Verification items for the finished model (mm, model axes). Face numbers are marked on the shaded views. A direction names the side the tool comes from. Round coordinates to 2 decimals unless told otherwise and drop trailing zeros. Write each loop counter-clockwise with the first axis right and the second up, starting at its lowest first coordinate (ties: lowest second). Pieces come first, ordered by that corner, then holes. Notation, with made-up numbers: (4, -1) - (49, -1) arc R28 ccw to (49, 17) - close; hole circle Ø11 at (-3.75, 4). An arc over 180 degrees is marked (long way). Answer as a JSON object with one key per item and string values. Group by question number.
1) Thickness scan on line 1 (Y direction, x = 0, z = -24.25); line 2 (Y direction, x = 3, z = -19.5); line 3 (Z direction, x = 3.5, y = -6.25). Record the ranges inside material, lowest first.
2) Section check B-B (z = 10). Enter the section's corners in (x, y).
3) Section check A-A (z = -29). Enter the section's corners in (x, y).
4) Section check C-C (x = -10.25). Enter the section's corners in (y, z), then the cut area to 3 significant figures.
5) Go/stop test with flat-tipped pins: pin 1 Ø12 at (x, z) = (-4, 14) entering from -Y; pin 2 Ø2 at (x, z) = (-1, -23.5) entering from -Y; pin 3 Ø2 at (y, z) = (2, -6) entering from +X. Record where each tip stops, or that it passes through.
6) Section check D-D (y = 8.25). Enter the section's corners in (x, z).
7) Set-up check for the marked faces 1, 2 and 3: record each of +Z, -Z, +X, -X, +Y, -Y from which the full face is reachable in a straight line by a thin tool's end or side.
```python
from build123d import *

# Parameters (mm, degrees)
SKETCH_1_R          = 6
EXTRUDE_1_DEPTH     = 20
EXTRUDE_2_DEPTH     = 6
SKETCH_3_R          = 7.5
EXTRUDE_3_DEPTH     = 1.5
SKETCH_4_R          = 5
EXTRUDE_4_DEPTH     = 26.5
SKETCH_6_R          = 6
SKETCH_6_R_2        = 5.5
CUT_EXTRUDE_1_DEPTH = 1
M5X0_8_1_D          = 4.2
M5X0_8_1_DEPTH      = 12.4
M5X0_8_1_TIP        = 1.2618073
CHAMFER_1_SIZE      = 1


with BuildPart() as part:
    # 草图1 → 凸台-拉伸1 (new body)
    with BuildSketch(Plane.XY):
        Circle(SKETCH_1_R)
    extrude(amount=EXTRUDE_1_DEPTH)

    # 草图2 → 凸台-拉伸2 (add)
    with BuildSketch(Plane(origin=(0, 0, 0), x_dir=(-1, 0, 0), z_dir=(0, 0, -1))):
        Polygon((6.350852961, 11), (-6.350852961, 11), (-12.701705922, 0), (-6.350852961, -11), (6.350852961, -11), (12.701705922, 0), align=None)
    extrude(amount=EXTRUDE_2_DEPTH)

    # 草图3 → 凸台-拉伸3 (add)
    with BuildSketch(Plane(origin=(0, 0, -6), x_dir=(-1, 0, 0), z_dir=(0, 0, -1))):
        Circle(SKETCH_3_R)
    extrude(amount=EXTRUDE_3_DEPTH)

    # 草图4 → 凸台-拉伸4 (add)
    with BuildSketch(Plane(origin=(0, 0, -7.5), x_dir=(-1, 0, 0), z_dir=(0, 0, -1))):
        Circle(SKETCH_4_R)
    extrude(amount=EXTRUDE_4_DEPTH)

    # 草图6 → 切除-拉伸1 (cut)
    with BuildSketch(Plane.XY):
        Circle(SKETCH_6_R)
        Circle(SKETCH_6_R_2, mode=Mode.SUBTRACT)
    extrude(amount=CUT_EXTRUDE_1_DEPTH, mode=Mode.SUBTRACT)

    # M5x0.8 螺纹孔1
    with Locations(Plane(origin=(0, 0, -34), x_dir=(-1, 0, 0), z_dir=(0, 0, -1))):
        with Locations((0, 0)):
            Hole(M5X0_8_1_D / 2, depth=M5X0_8_1_DEPTH)
            with Locations((0, 0, -(M5X0_8_1_DEPTH + M5X0_8_1_TIP / 2))):  # 118° drill point
                Cone(0, M5X0_8_1_D / 2, M5X0_8_1_TIP, mode=Mode.SUBTRACT)

    # 倒角1
    chamfer_1_edges = [part.edges().sort_by_distance(p)[0] for p in [
        (5, 0, -34),
        (-6, 0, 20),
    ]]
    chamfer(chamfer_1_edges, length=CHAMFER_1_SIZE)


solid = part.part
```
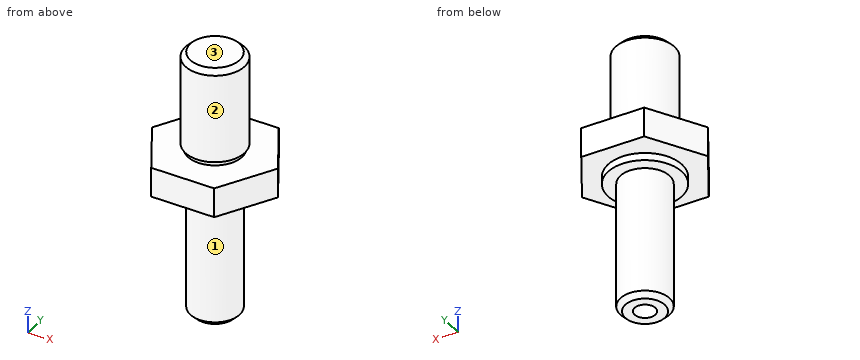
Returned:
{
 "1": {"line 1": "-5 to -2.1, 2.1 to 5", "line 2": "-4 to 4", "line 3": "-7.5 to 0"},
 "2": {"outline": "circle Ø12 at (0, 0)"},
 "3": {"outline": "circle Ø10 at (0, 0); hole circle Ø4.2 at (0, 0)"},
 "4": {"outline": "(-4.25, -6) - (4.25, -6) - (4.25, 0) - (-4.25, 0) - close", "area": "51.0 mm2"},
 "5": {"pin 1": "y = -6", "pin 2": "y = -5", "pin 3": "x = 12.12"},
 "6": {"outline": "(-7.94, -6) - (7.94, -6) - (7.94, 0) - (-7.94, 0) - close"},
 "7": {"face 1": "-Z", "face 2": "+Z", "face 3": "+Z, +X, -X, +Y, -Y"}
}
